Study the drawing (mm; zero at the part's minimum x, y, z) and answer. Round coordinates to 2 decimals unless told otherwise and drop trailing zeros. Order: outer loops, then holes, each group sorted by start corner. A loop starts at its lowest first (then second) coordinate and runs counter-clockwise, first axis right, second up. Notation, with made-up numbers: (-17, -20) - (39, -20) arc R19 cw to (39, -1) - close; hole circle Ø6 at (5, 80). An arc over 180 degrees is marked (long way). Put each result on its own line as item: value. Start each with the question number.
Q1. Find the intervals of material crossed by line 1 along X through (y, z) = (20, 25) (1 decimal); line 2 along Z through (x, y) = (32, 8); line 3 along X through (y, z) = (14, 23) (1 decimal), in increasing order. Write a range as from..to.
Q2. Each of these flat-tipped pins is pushed along its axis until it touches: pin 1 Ø3.5 at (x, z) = (17.46, 22.23) entering from -Y; pin 2 Ø3.5 at (x, z) = (17.46, 22.23) entering from +Y; pin 3 Ø4 at (x, y) = (24.61, 29.84) entering from -Z. Where does it stop, or does it pass through?
Q3. Section B-B on z = 28.5 is taken. Give the vertices of the cut face in (x, y) (1 decimal).
Q4. Section C-C on z = 5.5 is taken. Give the vertices of the cut face in (x, y) (1 decimal), then the cut area to 3 significant figures.
Q5. For a pull along X with two mould halves and no side action, classify the marked faces 1, 2 and 3 as pulls with the +X half, pulls with the -X half, needs draft (parallel to the pull), parting line crosses it, or undercut.
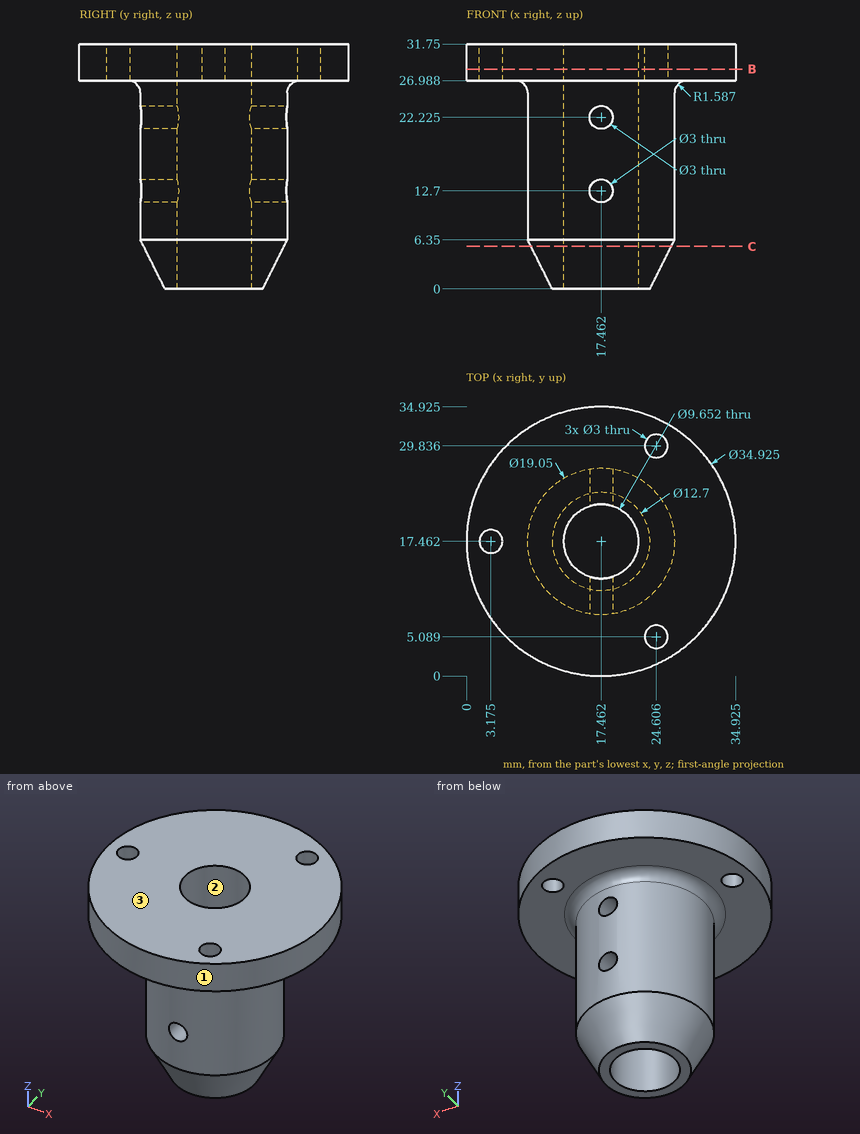
Findings:
1. line 1: 8.3..13.4, 21.6..26.6
1. line 2: 26.99..31.75
1. line 3: 8.6..14.1, 20.8..26.3
2. pin 1: y = 7.94
2. pin 2: y = 26.99
2. pin 3: z = 26.99
3. outline: circle Ø34.9 at (17.5, 17.5); hole circle Ø3 at (3.2, 17.5); hole circle Ø9.7 at (17.5, 17.5); hole circle Ø3 at (24.6, 5.1); hole circle Ø3 at (24.6, 29.8)
4. outline: circle Ø18.2 at (17.5, 17.5); hole circle Ø9.7 at (17.5, 17.5)
4. area: 187 mm2
5. face 1: parting line crosses it
5. face 2: undercut
5. face 3: needs draft
